```python
from build123d import *


# Not quite as in the source:
# - a fillet or chamfer that OpenCascade refuses, or shapes differently, is made with other operations: its cross-section is extruded or revolved along the edge and cut away or added


with BuildPart() as f1:
    # F0 (on Front) → F1 (revolve)
    with BuildSketch(Plane.XZ):
        with BuildLine():
            Line((0, 3.2086027786), (0, 0))
            Line((0, 0), (22.5, 0))
            Line((22.5, 0), (22.5, 1.1))
            ThreePointArc((22.5, 1.1), (20.1, 3.5), (22.5, 5.9))
            Line((22.5, 5.9), (22.5, 7))
            Line((22.5, 7), (3.9362940006, 7))
            Line((3.9362940006, 7), (3.9362940006, 10.5700949207))
            Line((3.9362940006, 10.5700949207), (1.281605335, 10.5700949207))
            Line((1.281605335, 10.5700949207), (1.281605335, 3.2086027786))
            Line((1.281605335, 3.2086027786), (0, 3.2086027786))
        make_face()
    revolve(axis=Axis((0, 0, 5.2850474603), (0, 0, -1)))

    # F2: fillet of radius 5 on 1 edges, made by hand

    # F2_s1 → F2_t2 (revolve)
    with BuildSketch(Plane.XZ):
        with BuildLine():
            ThreePointArc((8.7274704182, 7), (5.739956853, 7.9906655542), (3.9362940006, 10.5700949207))
            Line((3.9362940006, 10.5700949207), (3.9362940006, 7))
            Line((3.9362940006, 7), (8.7274704182, 7))
        make_face()
    revolve(axis=Axis((0, 0, 7), (0, 0, -1)))


solid = f1.part
```
Could you check a few things on this model? Use its own coordinates, in mm. A direction names the side the tool comes from. Round coordinates to 2 decimals unless told otherwise and drop trailing zeros. Write each loop counter-clockwise with the first axis right and the second up, starting at its lowest first coordinate (ties: lowest second). Pieces come first, ordered by that corner, then holes. Notation, with made-up numbers: M 33.5,58.5 L 47.5,58.5 A21 cw 47.5,68.5 Z; hole C -7.5,65 d7. An arc over 180 degrees is marked long. Write each question's results on one line, items separated by ' | '. Start each with the question number.
1. Thinking about a two-plate mould opening in X: for faces 1 (the face through (0, 10, 7)), 2 (the face through (0, 0, 3.209)), 3 (the face through (10.382, 19.961, 0.558)), which applies, +X half, -X half, draft (parallel to the pull), parting line (faces both ways), or undercut?
2. Imagine slicing it at C-C on z = 5.25. List the corners of the cut face in (x, y) for me, and give its area (3 significant figures).
3. Imagine slicing it at A-A on x = 0. List the corners of the cut face in (y, z) for me, and give its area (3 significant figures).
4. On a 3-axis mill with a long thin cutter (end or side, diameter ignored), from which of +Z, -Z, +X, -X, +Y, -Y can I reach the whole of each face in a straight line? I mean faces 4 (the face through (0, 0, 0)), 5 (the face through (-0.28, 1.25, 6.84)). Say none if no direction works.
5. I'm going to push flat-ended pins straight in: pin 1 Ø2 at (y, z) = (-16, 6.5) entering from +X; pin 2 Ø10 at (x, y) = (-16, 0.5) entering from +Z; pin 3 Ø5 at (x, z) = (5.5, 6.5) entering from +Y. Where does each tip first touch, or does it pass through?
6. I need wall thicknesses on L1, parallel to X at y = 0, z = 6; L2, parallel to Z at x = 13.5, y = -12.5; L3, parallel to Y at x = 0, z = 5.25. Which ranges of each line are inside material? Lowest first, please. Write a range as from..to.
Result sheet:
1) face 1: draft | face 2: undercut | face 3: parting line
2) outline: C 0,0 d41.72; hole C 0,0 d2.56 | area: 1,360 mm^2
3) outline: M -22.5,0 L 22.5,0 L 22.5,1.1 A2.4 cw 22.5,5.9 L 22.5,7 L 8.73,7 A5 cw 3.94,10.57 L 1.28,10.57 L 1.28,3.21 L -1.28,3.21 L -1.28,10.57 L -3.94,10.57 A5 cw -8.73,7 L -22.5,7 L -22.5,5.9 A2.4 cw -22.5,1.1 Z | area: 315 mm^2
4) face 4: -Z, +X, -X, +Y, -Y | face 5: +Z
5) pin 1: stops at x = 16.77 | pin 2: stops at z = 7 | pin 3: stops at y = 22.3
6) L1: x = -22.5..-1.28, 1.28..22.5 | L2: z = 0..7 | L3: y = -20.86..-1.28, 1.28..20.86
